The drawing under review shows one solid part. Ordinate dimensions are in mm from its lowest x, y, z. A direction names the side the tool comes from. Give positions to 0.01 mm unless a question says otherwise; leave off trailing zeros. Write each loop counter-clockwise with the first axis right and the second up, starting at its lowest first coordinate (ties: lowest second). Pieces come first, ordered by that corner, then holes. Notation, with made-up numbers: M 63,36.25 L 88,36.25 A23 ccw 88,47.25 Z; hole C -13,-10.5 d3. An arc over 180 degrees is marked long. Answer as a JSON object with one key per item and string values. Group by question number.
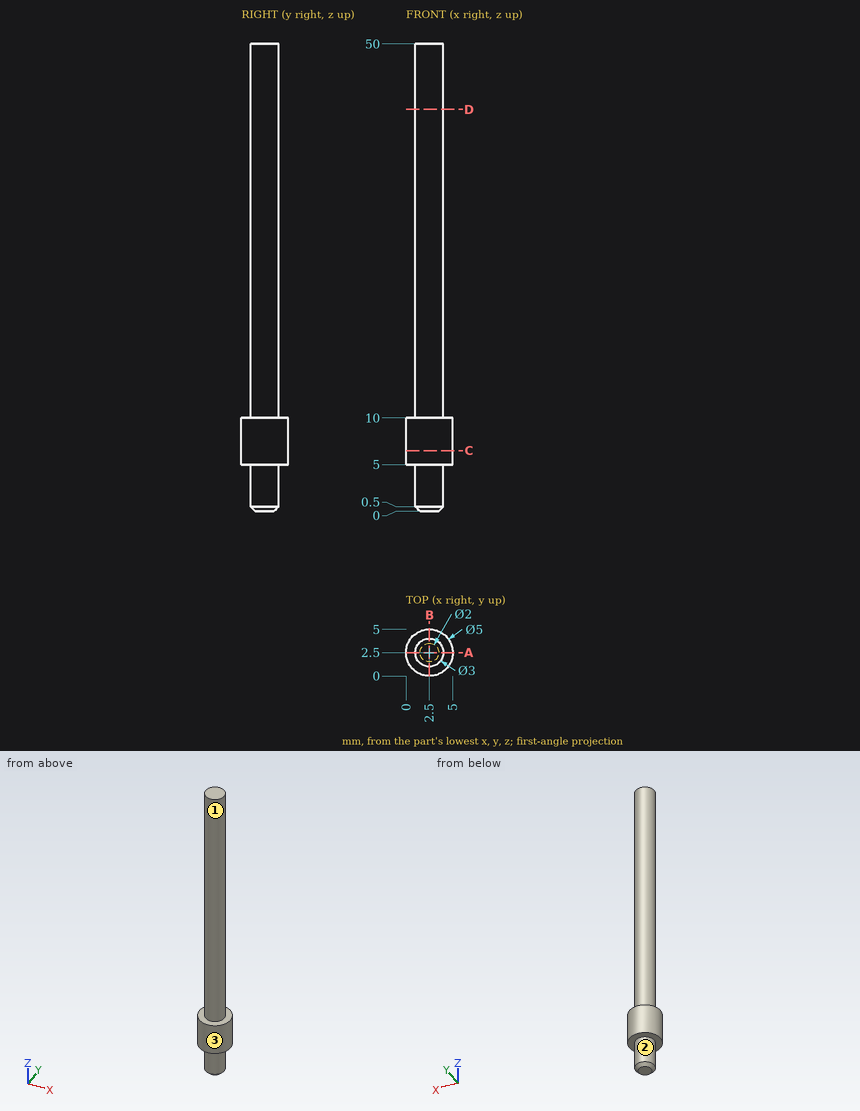
Item 1: Insertion check: P1, Ø2, axis at x = 3, z = 17.5, coming from the -Y side; P2, Ø1.5, axis at y = 4, z = 11.5, coming from the -X side; P3, Ø2, axis at x = 4.5, z = 25.5, coming from the +Y side. Each pin has a flat end and moves straight along its axis. Give the tip position at first contact, or say it passes through.
Item 2: Consider section D-D (z = 43). Give the boundary of the cut face in (x, y), plus the area to 3 significant figures.
Item 3: Machinability: for the marked faces 1, 2 and 3, which of the approach directions +Z, -Z, +X, -X, +Y, -Y give a long, thin tool a straight path to every point of the face, cutting with its end or side? Answer none if there is none.
Item 4: Consider section A-A (y = 2.5). Give the boundary of the cut face in (x, z), plus the area to 3 significant figures.
Item 5: Consider section C-C (z = 6.5). Give the boundary of the cut face in (x, y), plus the area to 3 significant figures.
Item 6: To check wall thickness, follow probe 1 along Z at (x, y) = (2.1, 4.3); probe 2 along Y at (x, z) = (2.6, 22); probe 3 along Z at (x, y) = (3.45, 3.3). State the ranges of each line that lie inside material, in increasing order.
Result set:
{
 "1": {"P1": "stops at y = 1", "P2": "stops at x = 1.2", "P3": "stops at y = 3.62"},
 "2": {"outline": "C 2.5,2.5 d3", "area": "7.07 mm^2"},
 "3": {"face 1": "+Z", "face 2": "-Z", "face 3": "+Z, -Z"},
 "4": {"outline": "M 0,5 L 1,5 L 1,0.5 L 1.5,0 L 3.5,0 L 4,0.5 L 4,5 L 5,5 L 5,10 L 4,10 L 4,50 L 1,50 L 1,10 L 0,10 Z", "area": "160 mm^2"},
 "5": {"outline": "C 2.5,2.5 d5", "area": "19.6 mm^2"},
 "6": {"probe 1": "z = 5 to 10", "probe 2": "y = 1 to 4", "probe 3": "z = 0.24 to 50"}
}
